Study the drawing (mm; zero at the part's minimum x, y, z) and answer. Coordinates: 2 decimals unless noted, no trailing zeros. Loops run counter-clockwise (first coordinate to the right, second up) from the corner with the lowest first, then second, coordinate; pieces in that order, holes last. Notation, with made-up numbers: (-31.5, -6) -> (-21.5, -6) arc R13 cw to (-21.5, 13) -> close; hole circle Ø6 at (-17, 39). An arc over 180 degrees is marked (long way). Answer in a Markdown table with one row per item.
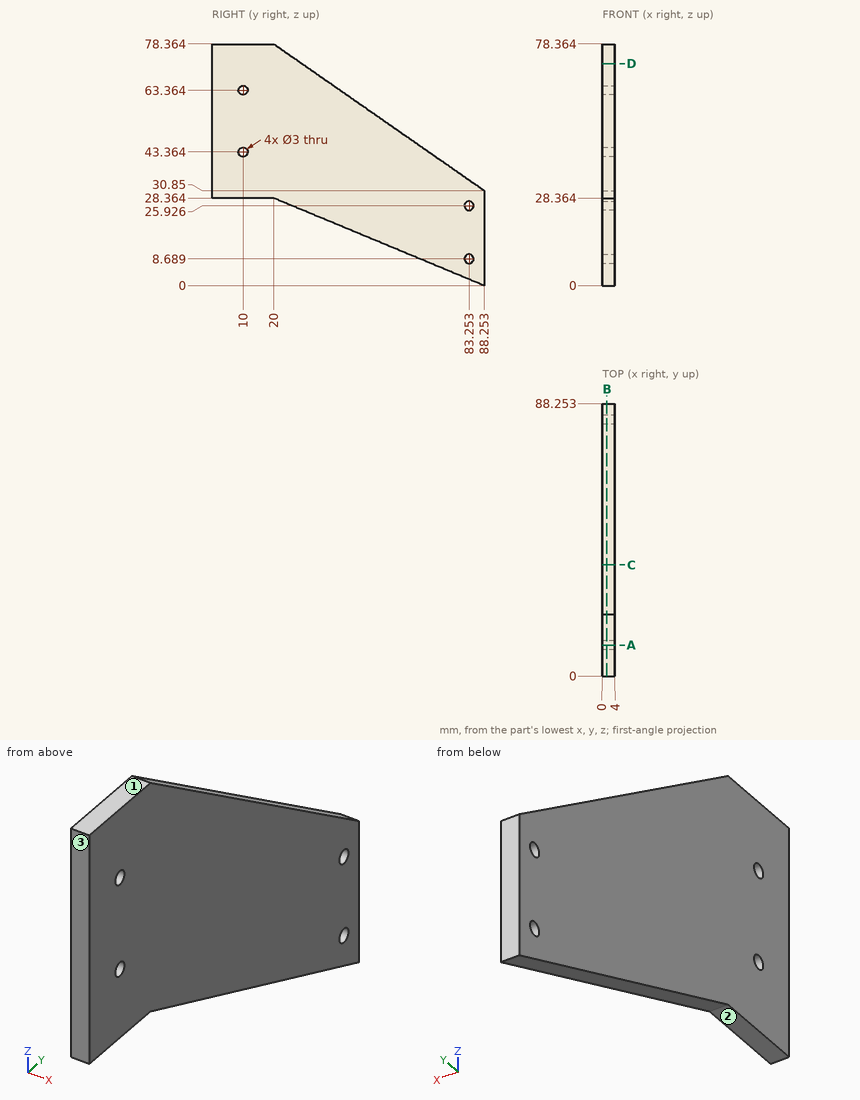
1. The mould has two halves that part along Z. Classify the marked faces 1, 2 and 3: pulls with the +Z half, pulls with the -Z half, needs draft (parallel to the pull), parting line crosses it, or undercut.
A:
| item | result |
|---|---|
| face 1 | pulls with the +Z half |
| face 2 | pulls with the -Z half |
| face 3 | needs draft |
2. A cutting plane is placed at C-C on y = 36. Give the vertices of the cut face in (x, z) (1 decimal), and give its area (3 significant figures).
A:
| item | result |
|---|---|
| outline | (0, 21.7) -> (4, 21.7) -> (4, 67.2) -> (0, 67.2) -> close |
| area | 182 mm2 |
3. A cutting plane is placed at B-B on x = 1.4. Give the vertices of the cut face in (y, z).
A:
| item | result |
|---|---|
| outline | (0, 28.36) -> (20, 28.36) -> (88.25, 0) -> (88.25, 30.85) -> (20, 78.36) -> (0, 78.36) -> close; hole circle Ø3 at (10, 43.36); hole circle Ø3 at (10, 63.36); hole circle Ø3 at (83.25, 8.69); hole circle Ø3 at (83.25, 25.93) |
4. A cutting plane is placed at D-D on z = 72. Give the vertices of the cut face in (x, y), and give its area (3 significant figures).
A:
| item | result |
|---|---|
| outline | (0, 0) -> (4, 0) -> (4, 29.14) -> (0, 29.14) -> close |
| area | 117 mm2 |
5. A cutting plane is placed at A-A on y = 10. Give the vertices of the cut face in (x, z), and give its area (3 significant figures).
A:
| item | result |
|---|---|
| outline | (0, 28.36) -> (4, 28.36) -> (4, 41.86) -> (0, 41.86) -> close; (0, 44.86) -> (4, 44.86) -> (4, 61.86) -> (0, 61.86) -> close; (0, 64.86) -> (4, 64.86) -> (4, 78.36) -> (0, 78.36) -> close |
| area | 176 mm2 |
6. Find the intervals of material crossed by probe 1 along Y at (x, z) = (0.65, 62.5) (1 decimal); probe 2 along Z at (x, y) = (3.35, 14); probe 3 along Z at (x, y) = (3, 84.5) (1 decimal), in increasing order.
A:
| item | result |
|---|---|
| probe 1 | y = 0 to 8.8, 11.2 to 42.8 |
| probe 2 | z = 28.36 to 78.36 |
| probe 3 | z = 1.6 to 7.9, 9.5 to 25.1, 26.8 to 33.5 |
7. Given pin 1 Ø1.5 at (x, y) = (1.5, 19.5) entering from -Z; pin 2 Ø1.5 at (x, y) = (1.5, 73.5) entering from -Z, each flat-ended and moving along its own axis, determine where each tip first touches the part or whether it passes through.
A:
| item | result |
|---|---|
| pin 1 | stops at z = 28.26 |
| pin 2 | stops at z = 5.82 |
